```python
from build123d import *

# Parameters (mm, degrees)
SKETCH_1_R          = 14
EXTRUDE_1_DEPTH     = 7
SKETCH_2_R          = 7.5
CUT_EXTRUDE_1_DEPTH = 8
SKETCH_3_R          = 12.65
SKETCH_3_R_2        = 9.4
CUT_EXTRUDE_2_DEPTH = 0.5
SKETCH_4_R          = 12.65
SKETCH_4_R_2        = 9.4
CUT_EXTRUDE_3_DEPTH = 0.5


with BuildPart() as part:
    # 草圖1 → 填料-伸長1 (new body)
    with BuildSketch(Plane.XY):
        Circle(SKETCH_1_R)
    extrude(amount=EXTRUDE_1_DEPTH)

    # 草圖2 → 除料-伸長1 (cut, through all)
    with BuildSketch(Plane.XY.offset(7)):
        Circle(SKETCH_2_R)
    extrude(amount=-CUT_EXTRUDE_1_DEPTH, mode=Mode.SUBTRACT)

    # 草圖3 → 除料-伸長2 (cut)
    with BuildSketch(Plane.XY.offset(7)):
        Circle(SKETCH_3_R)
        Circle(SKETCH_3_R_2, mode=Mode.SUBTRACT)
    extrude(amount=-CUT_EXTRUDE_2_DEPTH, mode=Mode.SUBTRACT)

    # 草圖4 → 除料-伸長3 (cut)
    with BuildSketch(Plane(origin=(0, 0, 0), x_dir=(-1, 0, 0), z_dir=(0, 0, -1))):
        Circle(SKETCH_4_R)
        Circle(SKETCH_4_R_2, mode=Mode.SUBTRACT)
    extrude(amount=-CUT_EXTRUDE_3_DEPTH, mode=Mode.SUBTRACT)


solid = part.part
```
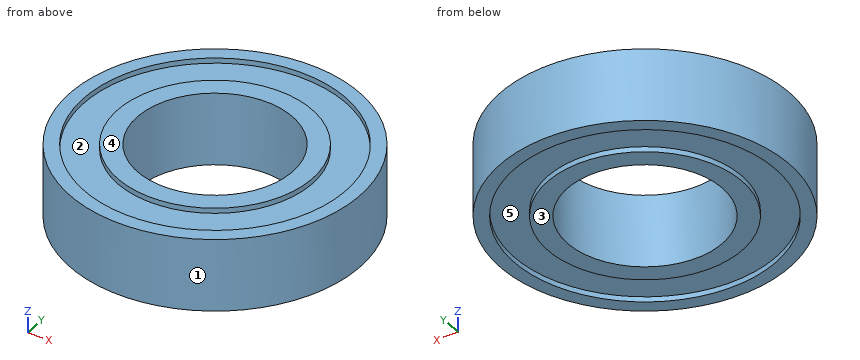
Model file for the job. Use its own axes, mm. Face numbers are marked on the shaded views. A direction names the side the tool comes from. Round coordinates to 2 decimals unless told otherwise and drop trailing zeros. Order: outer loops, then holes, each group sorted by start corner. A loop starts at its lowest first (then second) coordinate and runs counter-clockwise, first axis right, second up. Notation, with made-up numbers: (47, 33.5) -> (91, 33.5) arc R14 cw to (91, 42.5) -> close; hole circle Ø2 at (33.25, -13). An arc over 180 degrees is marked (long way). Use one line per item in the form item = value.
Item 1: Pull direction Y, two halves, no side cores. Call the marked faces 1, 2 and 3: released by +Y, released by -Y, zero draft, split by the parting line, or undercut.
Returned:
face_1 = split by the parting line
face_2 = undercut
face_3 = zero draft
Item 2: Cut at A-A, the plane y = 0. Write the cut outline in (x, z).
Returned:
outline = (-14, 0) -> (-12.65, 0) -> (-12.65, 0.5) -> (-9.4, 0.5) -> (-9.4, 0) -> (-7.5, 0) -> (-7.5, 7) -> (-9.4, 7) -> (-9.4, 6.5) -> (-12.65, 6.5) -> (-12.65, 7) -> (-14, 7) -> close; (7.5, 0) -> (9.4, 0) -> (9.4, 0.5) -> (12.65, 0.5) -> (12.65, 0) -> (14, 0) -> (14, 7) -> (12.65, 7) -> (12.65, 6.5) -> (9.4, 6.5) -> (9.4, 7) -> (7.5, 7) -> close
Item 3: Drill centre lines: line 1 (Y direction, x = 0, z = 0.2); line 2 (Y direction, x = 0, z = 5); line 3 (Z direction, x = -11.5, y = 4). Where is each one in solid material? Low to high.
Returned:
line_1 = -14 to -12.65, -9.4 to -7.5, 7.5 to 9.4, 12.65 to 14
line_2 = -14 to -7.5, 7.5 to 14
line_3 = 0.5 to 6.5
Item 4: Cut at D-D, the plane x = 10. Write the cut outline in (y, z).
Returned:
outline = (-9.8, 0) -> (-7.75, 0) -> (-7.75, 0.5) -> (7.75, 0.5) -> (7.75, 0) -> (9.8, 0) -> (9.8, 7) -> (7.75, 7) -> (7.75, 6.5) -> (-7.75, 6.5) -> (-7.75, 7) -> (-9.8, 7) -> close
Item 5: Flat gauge pins, fed straight in: pin 1 Ø5 at (x, y) = (-5.5, -2.5) entering from +Z; pin 2 Ø4 at (x, z) = (-10, 6) entering from -Y; pin 3 Ø12 at (x, y) = (0, 0) entering from +Z; pin 4 Ø2 at (x, z) = (8.5, 5) entering from +Y. Where does each tip first touch, or does it go through?
Returned:
pin_1 = 7
pin_2 = -11.49
pin_3 = through
pin_4 = 11.82
Item 6: Cut at C-C, the plane z = 2.5. Write the cut outline in (x, y).
Returned:
outline = circle Ø28 at (0, 0); hole circle Ø15 at (0, 0)
Item 7: Tool access for the marked faces 4 and 5: list every direction of +Z, -Z, +X, -X, +Y, -Y with a clear straight run to the whole face (end or side of a thin tool).
Returned:
face_4 = +Z, +X, -X, +Y, -Y
face_5 = -Z
